The listing builds one solid part. Answer for the finished solid, in the listing's coordinates (mm). Face numbers are marked on the shaded views. A direction names the side the tool comes from. Coordinates: 2 decimals unless noted, no trailing zeros. Loops run counter-clockwise (first coordinate to the right, second up) from the corner with the lowest first, then second, coordinate; pieces in that order, holes last. Notation, with made-up numbers: (1.25, 3) - (10.25, 3) arc R14 cw to (10.25, 29) - close; hole circle Ø1 at (-25.75, 25). An arc over 180 degrees is marked (long way). Write each question's results on one line, items separated by ' | '. Start each with the question number.
(1) Determine the mould class of the marked faces 1, 2 and 3 for opening direction Z: released by +Z, released by -Z, zero draft, split by the parting line, or undercut.
(2) Consider line 1 (Y direction, x = -3.5, z = 9); line 2 (X direction, y = 11, z = 7.25); line 3 (Z direction, x = 4.75, y = -3). Determine where each line is inside the solid, lowest interval first. Write a range as from..to.
(3) Find section B-B on x = 3. Determine the outline of the cut face in (y, z).
(4) For the marked faces 4, 5 and 6, determine the directions among +Z, -Z, +X, -X, +Y, -Y from which every point of the face is accessible in a straight line to the end or side of a thin tool.
(5) Given pin 1 Ø1.7 at (y, z) = (1.5, 9.5) entering from -X; pin 2 Ø1.5 at (y, z) = (9.5, 10.5) entering from -X; pin 3 Ø4 at (y, z) = (-0.5, 10.5) entering from -X, each flat-ended and moving along its own axis, determine where each tip first touches the part or whether it passes through.
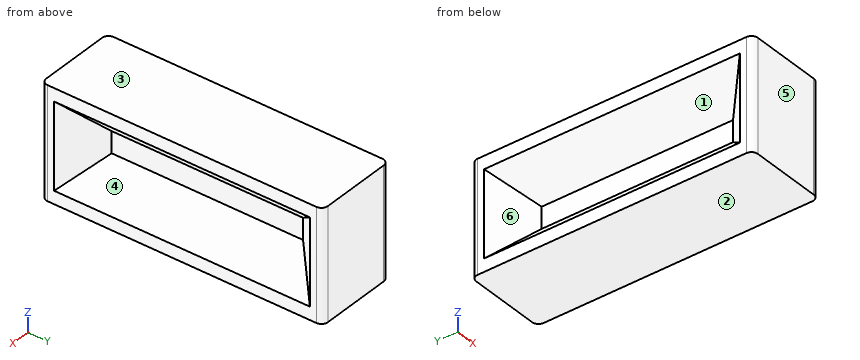
from build123d import *

# Parameters (mm, degrees)
F0_W     = 13
F0_H     = 43.7
F1_DEPTH = 17.3
F2_R     = 1
F3_W     = 39.7
F3_H     = 13.3
F5_DEPTH = 5
F4_W     = 39.7
F4_H     = 13.3
F6_DEPTH = 5
F7_SIZE  = 4.99999


# Not quite as in the source:
# - a fillet or chamfer is up to 0.001 mm smaller than in the source, because OpenCascade refuses the exact size


with BuildPart() as f1:
    # F0 (on Top) → F1 (new body)
    with BuildSketch(Plane.XY):
        Rectangle(F0_W, F0_H)
    extrude(amount=F1_DEPTH)

    # F2
    f2_edges = [f1.edges().sort_by_distance(p)[0] for p in [
        (-6.5, 21.85, 8.65),
        (6.5, 21.85, 8.65),
        (-6.5, -21.85, 8.65),
        (6.5, -21.85, 8.65),
    ]]
    fillet(f2_edges, radius=F2_R)

    # F3 (on face) → F5 (cut)
    with BuildSketch(Plane.YZ.offset(6.5)):
        with Locations((0, 8.65)):
            Rectangle(F3_W, F3_H)
    extrude(amount=-F5_DEPTH, mode=Mode.SUBTRACT)

    # F4 (on face) → F6 (cut)
    with BuildSketch(Plane(origin=(-6.5, 0, 0), x_dir=(0, -1, 0), z_dir=(-1, 0, 0))):
        with Locations((0, 8.65)):
            Rectangle(F4_W, F4_H)
    extrude(amount=-F6_DEPTH, mode=Mode.SUBTRACT)

    # F7 (size 5 in the source; OpenCascade refuses exactly that, so slightly less here)
    f7_edges = [f1.edges().sort_by_distance(p)[0] for p in [
        (-1.5, 0, 2),
        (-1.5, 19.85, 8.65),
        (-1.5, 0, 15.3),
        (-1.5, -19.85, 8.65),
        (1.5, 19.85, 8.65),
        (1.5, 0, 2),
        (1.5, -19.85, 8.65),
        (1.5, 0, 15.3),
    ]]
    chamfer(f7_edges, length=F7_SIZE)


solid = f1.part
Values:
1) face 1: undercut | face 2: released by -Z | face 3: released by +Z
2) line 1: y = -21.85..-16.85, 16.85..21.85 | line 2: x = -1.5..1.5 | line 3: z = 0..3.75, 13.55..17.3
3) outline: (-21.85, 0) - (21.85, 0) - (21.85, 17.3) - (-21.85, 17.3) - close; hole (-16.35, 5.5) - (16.35, 5.5) - (16.35, 11.8) - (-16.35, 11.8) - close
4) face 4: +X | face 5: +Z, -Z, +X, -X, -Y | face 6: -X
5) pin 1: stops at x = -1.55 | pin 2: stops at x = -2.45 | pin 3: stops at x = -3.7
